from build123d import *

# Parameters (mm, degrees)
F2_R     = 5.08
F4_R     = 7.62
F5_R     = 2.54
F6_R     = 4.7752
F7_DEPTH = 11.43
F8_R     = 1.6002
F9_DEPTH = 19.685


# Not quite as in the source:
# - a fillet or chamfer that OpenCascade refuses, or shapes differently, is made with other operations: its cross-section is extruded or revolved along the edge and cut away or added


with BuildPart() as f1:
    # F0 (on Front) → F1 (revolve)
    with BuildSketch(Plane.XZ):
        Polygon((0, 48.26), (0, 0), (5.4729898483, 5.3019602149), (28.3329898483, 5.3019602149), (28.3329898483, 30.7019602149), (17.0898887448, 30.7019602149), (17.0898887448, 38.7901112552), (10.16, 38.7901112552), (10.16, 48.26), align=None)
    revolve(axis=Axis((0, 0, 24.13), (0, 0, -1)))

    # F2
    f2_edges = [f1.edges().sort_by_distance(p)[0] for p in [
        (-17.089889, 0, 38.790111),
    ]]
    fillet(f2_edges, radius=F2_R)

    # F3: fillet of radius 12.7 on 1 edges, made by hand

    # F3_s1 → F3_t2 (revolve, cut)
    with BuildSketch(Plane.XZ):
        with BuildLine():
            ThreePointArc((17.0898887448, 30.7019602149), (25.1143562052, 26.5352808999), (28.3329898483, 18.085802099))
            Line((28.3329898483, 18.085802099), (28.3329898483, 30.7019602149))
            Line((28.3329898483, 30.7019602149), (17.0898887448, 30.7019602149))
        make_face()
    revolve(axis=Axis((0, 0, 30.7019602149), (0, 0, -1)), mode=Mode.SUBTRACT)

    # F4
    f4_edges = [f1.edges().sort_by_distance(p)[0] for p in [
        (-28.33299, 0, 5.30196),
    ]]
    fillet(f4_edges, radius=F4_R)

    # F5
    f5_edges = [f1.edges().sort_by_distance(p)[0] for p in [
        (-10.16, 0, 48.26),
    ]]
    fillet(f5_edges, radius=F5_R)

    # F6 (on face) → F7 (cut)
    with BuildSketch(Plane.XY.offset(48.26)):
        Circle(F6_R)
    extrude(amount=-F7_DEPTH, mode=Mode.SUBTRACT)

    # F8 (on Top) → F9 (cut)
    with BuildSketch(Plane.XY):
        Circle(F8_R)
    extrude(amount=F9_DEPTH, mode=Mode.SUBTRACT)


solid = f1.part
Model file for the job. Use its own axes, mm. A direction names the side the tool comes from. Round coordinates to 2 decimals unless told otherwise and drop trailing zeros. Loops run counter-clockwise (first coordinate to the right, second up) from the corner with the lowest first, then second, coordinate; pieces in that order, holes last. Notation, with made-up numbers: (72, 10) - (82, 10) arc R27 ccw to (82, 29) - close; hole circle Ø2 at (39.5, 16). An arc over 180 degrees is marked (long way). Write each question's results on one line, items separated by ' | '.
(1) Mould opens along Y. For faces 1 (the cylindrical face through (-6.14, 27.66, 15.54)), 2 (the flat face through (0, 5, 48.26)), 3 (the cylindrical face through (-1.27, -0.974, 10.491)), 4 (the cylindrical face through (-1.04, -4.66, 42.63)) say: released by +Y, released by -Y, zero draft, split by the parting line, or undercut.
Answer below:
face 1: split by the parting line | face 2: zero draft | face 3: undercut | face 4: undercut
(2) Saw through at D-D, the plane z = 22. List the corners of the cut face in (x, y), then the cut area to 3 significant figures.
Answer below:
outline: circle Ø55.43 at (0, 0) | area: 2,410 mm^2
(3) Pin check, flat tips, straight feed: pin 1 (12 mm diameter, centred on x = -8.5, y = -13, fed in from +Z); pin 2 (1 mm diameter, centred on x = -13, y = -22.5, fed in from +Z); pin 3 (5 mm diameter, centred on x = -10, z = 20.5, fed in from -Y). Stop position of each tip, or through.
Answer below:
pin 1: stops at z = 47.39 | pin 2: stops at z = 26.1 | pin 3: stops at y = -27.18
(4) Wall check: L1, parallel to Y at x = 0, z = 39.5; L2, parallel to Y at x = 0, z = 13.75; L3, parallel to Z at x = -6, y = 9. Give the ranges that are in metal, low to high.
Answer below:
L1: y = -10.16 to -4.78, 4.78 to 10.16 | L2: y = -28.33 to -1.6, 1.6 to 28.33 | L3: z = 5.3 to 38.79
(5) Saw through at C-C, the plane z = 44. List the corners of the cut face in (x, y), then the cut area to 3 significant figures.
Answer below:
outline: circle Ø20.32 at (0, 0); hole circle Ø9.55 at (0, 0) | area: 253 mm^2
(6) Saw through at A-A, the plane y = 0. List the corners of the cut face in (x, z) (3 decimals), then the cut area to 3 significant figures.
Answer below:
outline: (-28.333, 12.922) arc R7.62 ccw to (-20.713, 5.302) - (-5.473, 5.302) - (-1.6, 1.55) - (-1.6, 19.685) - (1.6, 19.685) - (1.6, 1.55) - (5.473, 5.302) - (20.713, 5.302) arc R7.62 ccw to (28.333, 12.922) - (28.333, 18.086) arc R12.7 ccw to (17.09, 30.702) - (17.09, 33.71) arc R5.08 ccw to (12.01, 38.79) - (10.16, 38.79) - (10.16, 45.72) arc R2.54 ccw to (7.62, 48.26) - (4.775, 48.26) - (4.775, 36.83) - (-4.775, 36.83) - (-4.775, 48.26) - (-7.62, 48.26) arc R2.54 ccw to (-10.16, 45.72) - (-10.16, 38.79) - (-12.01, 38.79) arc R5.08 ccw to (-17.09, 33.71) - (-17.09, 30.702) arc R12.7 ccw to (-28.333, 18.086) - close | area: 1,660 mm^2
(7) 3-axis set-ups, long thin cutter, end or side, ignore diameter. For faces 5 (the flat face through (0, 0, 36.83)), 6 (the flat face through (0, 0, 19.685)): which of +Z, -Z, +X, -X, +Y, -Y reach the whole face in a straight line?
Answer below:
face 5: +Z | face 6: -Z
